```python
from build123d import *

# Parameters (mm, degrees)
BOSS_EXTRUDE1_DEPTH                  = 5
BOSS_EXTRUDE1_DEPTH_BACK             = 5
SKETCH1_W                            = 100
SKETCH1_H                            = 100
SKETCH2_R                            = 7.5
SKETCH2_R_2                          = 3.25
CUT_EXTRUDE1_DEPTH                   = 12.7
TAP_DRILL_FOR_M5X0_8_TAP1_AT_2_COUNT = 2
TAP_DRILL_FOR_M5X0_8_TAP1_AT_2_PITCH = 70
SKETCH11_R                           = 37.5
CUT_EXTRUDE2_DEPTH                   = 3
CHAMFER1_SIZE                        = 0.5
SKETCH12_R                           = 1.75
CUT_EXTRUDE3_DEPTH                   = 72.414284285
SKETCH13_R                           = 2.25
CUT_EXTRUDE4_DEPTH                   = 10


with BuildPart() as part:
    # Sketch1 → Boss-Extrude1 (new, two sides: drawn at the far end of the back side and taken through both)
    with BuildSketch(Plane(origin=(0, 0, 0), x_dir=(1, 0, 0), z_dir=(0, 1, 0)).offset(-BOSS_EXTRUDE1_DEPTH_BACK)):
        Rectangle(SKETCH1_W, SKETCH1_H)
    extrude(amount=BOSS_EXTRUDE1_DEPTH + BOSS_EXTRUDE1_DEPTH_BACK)

    # Sketch2 → Cut-Extrude1 (cut)
    with BuildSketch(Plane(origin=(0, 5, 0), x_dir=(1, 0, 0), z_dir=(0, 1, 0))):
        with Locations(Location((0, 0, 0), (0, 0, 270))):
            Circle(SKETCH2_R)
        with Locations(Location((-34.798492469, 34.798492469, 0), (0, 0, 270))):
            Circle(SKETCH2_R_2)
        with Locations(Location((34.798492469, 34.798492469, 0), (0, 0, 270))):
            Circle(SKETCH2_R_2)
        with Locations(Location((34.798492469, -34.798492469, 0), (0, 0, 270))):
            Circle(SKETCH2_R_2)
        with Locations(Location((-34.798492469, -34.798492469, 0), (0, 0, 270))):
            Circle(SKETCH2_R_2)
    extrude(amount=-CUT_EXTRUDE1_DEPTH, mode=Mode.SUBTRACT)

    # Sketch10 → Tap Drill for M5x0.8 Tap1 (revolve, cut)
    with BuildSketch(Plane(origin=(-50, 0, -35), x_dir=(0, 0, 1), z_dir=(0, 1, 0))):
        Polygon((0, 0), (0, 11.2618073), (2.1, 10), (2.1, 0), align=None)
    tap_drill_for_m5x0_8_tap1 = revolve(axis=Axis((-56.35, 0, -35), (1, 0, 0)), mode=Mode.SUBTRACT)

    # Tap Drill for M5x0.8 Tap1 at 2: Tap Drill for M5x0.8 Tap1 ×2
    with Locations(*[(0, 0, i * TAP_DRILL_FOR_M5X0_8_TAP1_AT_2_PITCH) for i in range(1, TAP_DRILL_FOR_M5X0_8_TAP1_AT_2_COUNT)]):
        add(tap_drill_for_m5x0_8_tap1, mode=Mode.SUBTRACT)

    # Sketch11 → Cut-Extrude2 (cut)
    with BuildSketch(Plane.XZ.offset(5)):
        with Locations(Location((0, 0, 0), (0, 0, 270))):
            Circle(SKETCH11_R)
    extrude(amount=-CUT_EXTRUDE2_DEPTH, mode=Mode.SUBTRACT)

    # Chamfer1
    chamfer1_edges = [part.edges().sort_by_distance(p)[0] for p in [
        (-50, 0, -50),
        (50, 0, -50),
        (50, 0, 50),
        (-50, 0, 50),
    ]]
    chamfer(chamfer1_edges, length=CHAMFER1_SIZE)

    # Mirror1: Tap Drill for M5x0.8 Tap1 across plane
    add(tap_drill_for_m5x0_8_tap1.mirror(Plane.ZY), mode=Mode.SUBTRACT)

    # Mirror1 copy 1 sketch → Mirror1 copy 1 (revolve, cut)
    with BuildSketch(Plane(origin=(50, 0, 35), x_dir=(0, 0, 1), z_dir=(0, 1, 0))):
        Polygon((0, 0), (0, -11.2618073), (2.1, -10), (2.1, 0), align=None)
    revolve(axis=Axis((56.35, 0, 35), (1, 0, 0)), mode=Mode.SUBTRACT)

    # Sketch12 → Cut-Extrude3 (cut, through all)
    with BuildSketch(Plane(origin=(0, 5, 0), x_dir=(1, 0, 0), z_dir=(0, 1, 0))):
        with Locations(Location((7.75, 20.423393759, 0), (0, 0, 270))):
            Circle(SKETCH12_R)
        with Locations(Location((-7.75, 20.423393759, 0), (0, 0, 270))):
            Circle(SKETCH12_R)
        with Locations(Location((15.5, 7, 0), (0, 0, 90))):
            Circle(SKETCH12_R)
        with Locations(Location((7.75, -6.423393759, 0), (0, 0, 270))):
            Circle(SKETCH12_R)
        with Locations(Location((-7.75, -6.423393759, 0), (0, 0, 270))):
            Circle(SKETCH12_R)
        with Locations(Location((-15.5, 7, 0), (0, 0, 270))):
            Circle(SKETCH12_R)
    extrude(amount=-CUT_EXTRUDE3_DEPTH, mode=Mode.SUBTRACT)

    # Sketch13 → Cut-Extrude4 (cut)
    with BuildSketch(Plane(origin=(0, 5, 0), x_dir=(1, 0, 0), z_dir=(0, 1, 0))):
        with Locations(Location((-15.5, -15.5, 0), (0, 0, 270))):
            Circle(SKETCH13_R)
        with Locations(Location((-15.5, 15.5, 0), (0, 0, 270))):
            Circle(SKETCH13_R)
        with Locations(Location((15.5, 15.5, 0), (0, 0, 270))):
            Circle(SKETCH13_R)
        with Locations(Location((15.5, -15.5, 0), (0, 0, 270))):
            Circle(SKETCH13_R)
    extrude(amount=-CUT_EXTRUDE4_DEPTH, mode=Mode.SUBTRACT)


solid = part.part
```
The model under review builds one solid part; all positions refer to its coordinate system, in mm. A direction names the side the tool comes from. Round coordinates to 2 decimals unless told otherwise and drop trailing zeros. Loops run counter-clockwise (first coordinate to the right, second up) from the corner with the lowest first, then second, coordinate; pieces in that order, holes last. Notation, with made-up numbers: (63, 86.25) - (78, 86.25) arc R18 cw to (78, 100.25) - close; hole circle Ø1 at (41, 66.5). An arc over 180 degrees is marked (long way). Write each question's results on one line, items separated by ' | '. Start each with the question number.
Q1. Insertion check: P1, Ø5, axis at x = 4, z = -26.5, coming from the -Y side; P2, Ø3, axis at x = 15.5, z = -7, coming from the +Y side; P3, Ø2.5, axis at y = 0, z = -35, coming from the -X side. Each pin has a flat end and moves straight along its axis. Give the tip position at first contact, or say it passes through.
Q2. Take a section at B-B on z = 15.5. Give the boundary of the cut face in (x, y).
Q3. Wall thickness on line 1 along Z through (x, y) = (-47, 0); line 2 along Z through (x, y) = (-35.5, 4): over which ranges is each line inside the solid? List them lowest first. Write a range as [from, to].
Q4. Take a section at D-D on x = 26. Give the boundary of the cut face in (y, z).
Q5. Draft analysis for pull direction Y (two halves, no side actions). For faces 4 (the cylindrical face through (-45.07, -0.09, 32.9)), 5 (the cylindrical face through (-9.303, 1.549, 7.231)), 6 (the flat face through (-23, -5, -34)), state which applies: pulls with the +Y half, pulls with the -Y half, needs draft (parallel to the pull), parting line crosses it, or undercut.
Q6. Tool access review of faces 1 (the cylindrical face through (45.07, -0.09, -37.1)), 2 (the cylindrical face through (-22.818, -3.521, 29.759)), 3 (the flat face through (50, 0, 1)): name each direction out of +Z, -Z, +X, -X, +Y, -Y from which nothing blocks a thin tool from reaching the whole face with its end or side.
Q7. Take a section at C-C on x = 15.5. Give the boundary of the cut face in (y, z).
Q8. Take a section at A-A on x = 0. Give the boundary of the cut face in (y, z), plus the area to 3 significant figures.
Data:
1) P1: stops at y = -2 | P2: passes through | P3: stops at x = -39.49
2) outline: (-50, -5) - (-34.15, -5) - (-34.15, -2) - (-17.75, -2) - (-17.75, 5) - (-50, 5) - close; (-13.25, -2) - (13.25, -2) - (13.25, 5) - (-13.25, 5) - close; (17.75, -2) - (34.15, -2) - (34.15, -5) - (50, -5) - (50, 5) - (17.75, 5) - close
3) line 1: z = [-50, -37.1], [-32.9, 32.9], [37.1, 50] | line 2: z = [-50, -37.97], [-31.63, 31.63], [37.97, 50]
4) outline: (-5, -50) - (5, -50) - (5, 50) - (-5, 50) - (-5, 27.02) - (-2, 27.02) - (-2, -27.02) - (-5, -27.02) - close
5) face 4: undercut | face 5: needs draft | face 6: pulls with the -Y half
6) face 1: +X | face 2: -Y | face 3: +Z, -Z, +X, +Y, -Y
7) outline: (-5, -50) - (5, -50) - (5, -17.75) - (-2, -17.75) - (-2, -34.15) - (-5, -34.15) - close; (-5, 34.15) - (-2, 34.15) - (-2, 17.75) - (5, 17.75) - (5, 50) - (-5, 50) - close; (-2, -13.25) - (5, -13.25) - (5, -8.75) - (-2, -8.75) - close; (-2, -5.25) - (5, -5.25) - (5, 13.25) - (-2, 13.25) - close
8) outline: (-5, -50) - (5, -50) - (5, -7.5) - (-2, -7.5) - (-2, -37.5) - (-5, -37.5) - close; (-5, 37.5) - (-2, 37.5) - (-2, 7.5) - (5, 7.5) - (5, 50) - (-5, 50) - close | area: 670 mm²
